Geometry check sheet. Reference: the model listing, model coordinates, mm. A direction names the side the tool comes from. Coordinates: 2 decimals unless noted, no trailing zeros. Loops run counter-clockwise (first coordinate to the right, second up) from the corner with the lowest first, then second, coordinate; pieces in that order, holes last.
from build123d import *

# Parameters (mm, degrees)
ESQUISSE1_W             = 100
ESQUISSE1_H             = 100
BOSS_EXTRU_1_DEPTH      = 3
ESQUISSE2_W             = 10
ESQUISSE2_H             = 20
BOSS_EXTRU_2_DEPTH      = 10
CHANFREIN1_SIZE         = 10
ESQUISSE3_R             = 1.525
ENL_V_MAT_EXTRU_1_DEPTH = 118.3413823
CHANFREIN2_SIZE         = 3
ESQUISSE4_W             = 5
ESQUISSE4_H             = 10
BOSS_EXTRU_3_DEPTH      = 10
ESQUISSE5_R             = 1.75
ENL_V_MAT_EXTRU_2_DEPTH = 10
ESQUISSE6_W             = 55.202992824
ESQUISSE6_H             = 76.399934011
ENL_V_MAT_EXTRU_3_DEPTH = 10
ESQUISSE9_W             = 10
ESQUISSE9_H             = 5
BOSS_EXTRU_5_DEPTH      = 10
ESQUISSE10_R            = 1.75
ENL_V_MAT_EXTRU_5_DEPTH = 10
CHANFREIN3_SIZE         = 6


with BuildPart() as part:
    # Esquisse1 → Boss.-Extru.1 (new body)
    with BuildSketch(Plane.XY):
        with Locations((50, 50)):
            Rectangle(ESQUISSE1_W, ESQUISSE1_H)
    extrude(amount=BOSS_EXTRU_1_DEPTH)

    # Esquisse2 → Boss.-Extru.2 (add)
    with BuildSketch(Plane.XY.offset(3)):
        with Locations((5.05, 50)):
            Rectangle(ESQUISSE2_W, ESQUISSE2_H)
        with Locations((94.95, 50)):
            Rectangle(ESQUISSE2_W, ESQUISSE2_H)
    extrude(amount=BOSS_EXTRU_2_DEPTH)

    # Chanfrein1
    chanfrein1_edges = [part.edges().sort_by_distance(p)[0] for p in [
        (94.95, 60, 13),
        (5.05, 60, 13),
    ]]
    chamfer(chanfrein1_edges, length=CHANFREIN1_SIZE - 0.0001)  # a hair under: the kernel refuses the full size

    # Esquisse3 → Enlèv. mat.-Extru.1 (cut, through all)
    with BuildSketch(Plane.XZ.offset(-40)):
        with Locations(Location((5.046227865, 8, 0), (0, 0, 270))):
            Circle(ESQUISSE3_R)
        with Locations(Location((94.95, 8, 0), (0, 0, 270))):
            Circle(ESQUISSE3_R)
    extrude(amount=-ENL_V_MAT_EXTRU_1_DEPTH, mode=Mode.SUBTRACT)

    # Chanfrein2
    chanfrein2_edges = [part.edges().sort_by_distance(p)[0] for p in [
        (50, 0, 0),
        (100, 50, 0),
        (50, 100, 0),
        (0, 50, 0),
    ]]
    chamfer(chanfrein2_edges, length=CHANFREIN2_SIZE - 0.0001)  # a hair under: the kernel refuses the full size

    # Esquisse4 → Boss.-Extru.3 (add)
    with BuildSketch(Plane.XY.offset(3)):
        with Locations((62.5, 94.95)):
            Rectangle(ESQUISSE4_W, ESQUISSE4_H)
    extrude(amount=BOSS_EXTRU_3_DEPTH)

    # Esquisse5 → Enlèv. mat.-Extru.2 (cut)
    with BuildSketch(Plane(origin=(65, 0, 0), x_dir=(0, 0, -1), z_dir=(1, 0, 0))):
        with Locations((-8.05, 94.95)):
            Circle(ESQUISSE5_R)
    extrude(amount=-ENL_V_MAT_EXTRU_2_DEPTH, mode=Mode.SUBTRACT)

    # Esquisse6 → Enlèv. mat.-Extru.3 (cut)
    with BuildSketch(Plane.XY.offset(3)):
        with Locations((87.601496412, 31.800032995)):
            Rectangle(ESQUISSE6_W, ESQUISSE6_H)
    extrude(amount=-ENL_V_MAT_EXTRU_3_DEPTH, mode=Mode.SUBTRACT)


with BuildPart() as body_2:
    # of the pieces the cut leaves, the one that is kept (enl_v_mat_extru_3_keep)
    add(part.part.solids().sort_by_distance((0, 100, 2.9999))[0])

    # Esquisse9 → Boss.-Extru.5 (add)
    with BuildSketch(Plane.XY.offset(3)):
        with Locations((94.95, 72.55)):
            Rectangle(ESQUISSE9_W, ESQUISSE9_H)
    extrude(amount=BOSS_EXTRU_5_DEPTH)

    # Esquisse10 → Enlèv. mat.-Extru.5 (cut)
    with BuildSketch(Plane.XZ.offset(-70)):
        with Locations(Location((94.95, 8, 0), (0, 0, 270))):
            Circle(ESQUISSE10_R)
    extrude(amount=-ENL_V_MAT_EXTRU_5_DEPTH, mode=Mode.SUBTRACT)

    # Chanfrein3
    chanfrein3_edges = [body_2.edges().sort_by_distance(p)[0] for p in [
        (60, 70, 1.5),
    ]]
    chamfer(chanfrein3_edges, length=CHANFREIN3_SIZE)


solid = body_2.part
(1) Gauge pin test, flat ends, axial feed: pin 1 Ø2.5 at (y, z) = (73.5, 6) entering from -X; pin 2 Ø1.5 at (x, z) = (62, 8.5) entering from +Y; pin 3 Ø1.5 at (x, z) = (62, 7.5) entering from -Y. Record the tip position at first contact, or that the pin passes through.
Findings:
pin 1: stops at x = 89.95
pin 2: stops at y = 99.95
pin 3: stops at y = 89.95
(2) Scan lines: L1, parallel to X at y = 73.75, z = 8; L2, parallel to X at y = 44.75, z = 8; L3, parallel to Z at x = 62.3, y = 94.95. Record each from-to range of solid material in increasing order.
Findings:
L1: x = 89.95 to 93.2, 96.7 to 99.95
L2: x = 0.05 to 3.52, 6.57 to 10.05
L3: z = 0 to 6.3, 9.8 to 13
(3) Sectioned sample at D-D on z = 8.05. Record the cut outline in (x, y).
Findings:
outline: (0.05, 40) - (3.52, 40) - (3.52, 54.95) - (0.05, 54.95) - close; (6.57, 40) - (10.05, 40) - (10.05, 54.95) - (6.57, 54.95) - close; (60, 89.95) - (65, 89.95) - (65, 93.2) - (60, 93.2) - close; (60, 96.7) - (65, 96.7) - (65, 99.95) - (60, 99.95) - close; (89.95, 70.05) - (93.2, 70.05) - (93.2, 75.05) - (89.95, 75.05) - close; (96.7, 70.05) - (99.95, 70.05) - (99.95, 75.05) - (96.7, 75.05) - close
(4) Access from +Z, -Z, +X, -X, +Y, -Y to the whole of each face (thin tool, end or side, straight path). Record for faces 1 (the flat face through (93, 75.05, 8)), 2 (the flat face through (62, 89.95, 8)), 3 (the flat face through (65, 93, 8)).
Findings:
face 1: +Z, +X, -X, +Y
face 2: +Z, +X, -X, -Y
face 3: +Z, +X, +Y, -Y
